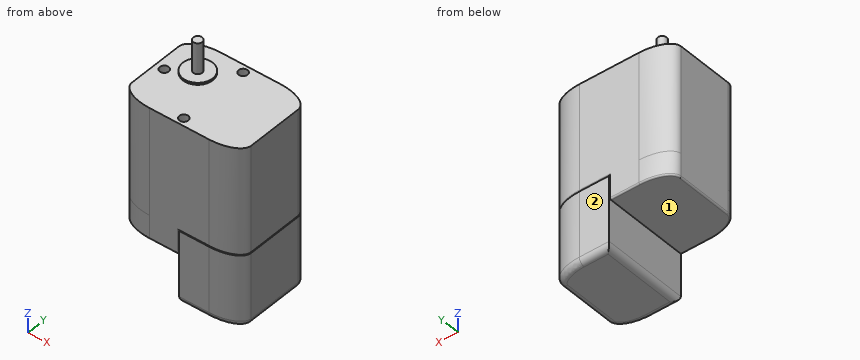
Autodesk Inventor part; units mm, degrees
ref_plane "YZ Plane" through (0, 0, 0) normal (1, 0, 0) x (0, 1, 0)
ref_plane "XZ Plane" through (0, 0, 0) normal (0, 1, 0) x (-1, 0, 0)
ref_plane "XY Plane" through (0, 0, 0) normal (0, 0, 1) x (1, 0, 0)
sketch "Sketch1" plane through (0, 0, 0) normal (0, 0, 1) x (1, 0, 0)
  ellipse E0 centre (10, 24) end of major axis (0, 24) minor radius 5 (10, 29) -> (0, 24) ccw
  ellipse E1 centre (30, 24) end of major axis (40, 24) minor radius 5 (40, 24) -> (30, 29) ccw
  ellipse E2 centre (30, 5) end of major axis (40, 5) minor radius 5 (30, 0) -> (40, 5) ccw
  ellipse E3 centre (10, 5) end of major axis (0, 5) minor radius 5 (0, 5) -> (10, 0) ccw
  line L0 (30, 29) -> (10, 29)
  line L1 (0, 24) -> (0, 5)
  line L2 (10, 0) -> (30, 0)
  line L3 (40, 5) -> (40, 24)
  point P0 (0, 0)
extrude "Extrusion2" add sketch "Sketch1" along normal blind 36
sketch "Sketch2" plane through (0, 0, 36) normal (0, 0, 1) x (1, 0, 0)
  line L0 (0, 24) -> (0, 5)
  line L1 (10, 0) -> (30, 0)
  line L2 (30, 29) -> (10, 29)
  line L3 (14.358, 14.5) -> (-3.5199, 14.5)
  circle A0 centre (3, 14.5) radius 1.5
  line L4 (21.3512, 2.5) -> (5.4191, 2.5)
  line L5 (21.3512, 26.5) -> (5.4191, 26.5)
  line L6 (19.5, 31.1643) -> (19.5, -4.236)
  circle A1 centre (19.5, 26.5) radius 1.5001
  circle A2 centre (19.5, 2.5) radius 1.5001
  point P0 (0, 0)
  dimension "d16" = 29
  dimension "d17" = 14.5
  dimension "d18" = 3
  dimension "d19" = 3
  dimension "d20" = 24
  dimension "d21" = 12
  dimension "d22" = 16.5
extrude "Extrusion3" cut sketch "Sketch2" against normal blind 5
thread "Thread1"
thread "Thread2"
thread "Thread3"
sketch "Sketch3" plane through (0, 0, 36) normal (0, 0, 1) x (1, 0, 0)
  line L0 (0, 24) -> (0, 5)
  line L1 (30, 29) -> (10, 29)
  line L2 (-1.3483, 17.5) -> (17.9999, 17.5)
  line L3 (12, 35.2177) -> (12, 13)
  circle A0 centre (10.5, 19) radius 1.5
  point P0 (0, 0)
  dimension "d31" = 11.5
  dimension "d32" = 12
  dimension "d33" = 3
  dimension "d34" = 1.5
  dimension "d35" = 1.5
extrude "Extrusion4" add sketch "Sketch3" along normal blind 11 contours A0
sketch "Sketch4" plane through (0, 0, 36) normal (0, 0, 1) x (1, 0, 0)
  circle A0 centre (10.5, 19) radius 1.5
  circle A1 centre (10.5, 19) radius 5
  point P0 (0, 0)
  dimension "d40" = 10
extrude "Extrusion5" add sketch "Sketch4" along normal blind 0.67
sketch "Sketch5" plane through (0, 0, 0) normal (0, 0, -1) x (-1, 0, 0)
  ellipse E0 centre (-10, 24) end of major axis (0, 24) minor radius 5 (0, 24) -> (-10, 29) ccw
  line L0 (-30, 29) -> (-10, 29)
  line L1 (-40, 5) -> (-40, 24)
  line L2 (-10, 0) -> (-30, 0)
  ellipse E1 centre (-10, 5) end of major axis (0, 5) minor radius 5 (-10, 0) -> (0, 5) ccw
  line L3 (0, 24) -> (0, 5)
  line L4 (-20, 29) -> (-20, 0)
  point P0 (0, 0)
  dimension "d42" = 40
  dimension "d43" = 20
extrude "Extrusion6" add sketch "Sketch5" along normal blind 8
sketch "Sketch6" plane through (0, 0, 0) normal (0, 0, -1) x (-1, 0, 0)
  line L0 (-20, 0) -> (-20, 29)
  line L1 (-30, 29) -> (-20, 29)
  ellipse E0 centre (-30, 24) end of major axis (-40, 24) minor radius 5 (-30, 29) -> (-40, 24) ccw
  line L2 (-40, 5) -> (-40, 24)
  ellipse E1 centre (-30, 5) end of major axis (-40, 5) minor radius 5 (-40, 5) -> (-30, 0) ccw
  line L3 (-20, 0) -> (-30, 0)
  point P0 (0, 0)
fillet "Fillet2" radius 0.5 13 edges at (15, 29, -8) (0, 14.5, -8) (2.9289, 1.4645, -8) (15, 0, -8) (2.9289, 27.5355, -8) (20, 29, -4) (37.0711, 27.5355, 0) (40, 14.5, 0) (37.0711, 1.4645, 0) (25, 0, 0) (25, 29, 0) (20, 14.5, -8) (20, 0, -4)
extrude "Extrusion8" add sketch "Sketch6" along normal blind 24
fillet "Fillet3" radius 2 6 edges at (25, 0, -24) (40, 14.5, -24) (37.0711, 27.5355, -24) (25, 29, -24) (37.0711, 1.4645, -24) (20, 14.5, -24)
properties part number "12V geared motor"
Could you check a few things on this model? Use its own coordinates, in mm. Face numbers are marked on the shaded views. A direction names the side the tool comes from. Coordinates: 2 decimals unless noted, no trailing zeros. Loops run counter-clockwise (first coordinate to the right, second up) from the corner with the lowest first, then second, coordinate; pieces in that order, holes last.
1) Will these pins go through, and if not, where does the flat tip stop? pin 1 Ø5 at (x, y) = (3, 14.5) entering from +Z; pin 2 Ø1 at (x, z) = (31.5, 12.5) entering from +Y; pin 3 Ø1 at (x, y) = (17.5, 6.5) entering from -Z.
Reported:
pin 1: stops at z = 36
pin 2: stops at y = 28.97
pin 3: stops at z = -8
2) Imagine slicing it at D-D (y = 22.5). List the corners of the cut face in (x, z) for me.
Reported:
outline: (0, -7.5) arc R0.5 ccw to (0.5, -8) - (19.5, -8) arc R0.5 ccw to (20, -7.5) - (20, -22) arc R2 ccw to (22, -24) - (38, -24) arc R2 ccw to (40, -22) - (40, 0) - (39.5, 0) arc R0.5 ccw to (40, 0.5) - (40, 36) - (14.07, 36) - (14.07, 36.67) - (6.93, 36.67) - (6.93, 36) - (0, 36) - close
3) Imagine slicing it at B-B (x = 24). List the corners of the cut face in (y, z) for me.
Reported:
outline: (0, -22) arc R2 ccw to (2, -24) - (27, -24) arc R2 ccw to (29, -22) - (29, 0) - (28.5, 0) arc R0.5 ccw to (29, 0.5) - (29, 36) - (0, 36) - (0, 0.5) arc R0.5 ccw to (0.5, 0) - (0, 0) - close
4) Which directions (+Z, -Z, +X, -X, +Y, -Y) give clear straight access to the entire face, cutting with the end or side of a thin tool? Please do the marked faces 1 and 2.
Reported:
face 1: -Z, -X, +Y, -Y
face 2: +Z, -Z, +X, -X, +Y
5) Please list where these lines run through material, in increasing order: line 1 along Y through (x, z) = (19.5, 32.9); line 2 along X through (y, z) = (14.5, 33.9); line 3 along Z through (x, y) = (7, 13).
Reported:
line 1: y = 0 to 1, 4 to 25, 28 to 29
line 2: x = 0 to 1.5, 4.5 to 40
line 3: z = -8 to 36
6) Imagine slicing it at A-A (y = 9.5). List the corners of the cut face in (x, z) for me, and give its area (3 significant figures).
Reported:
outline: (0, -7.5) arc R0.5 ccw to (0.5, -8) - (19.5, -8) arc R0.5 ccw to (20, -7.5) - (20, -22) arc R2 ccw to (22, -24) - (38, -24) arc R2 ccw to (40, -22) - (40, 0) - (39.5, 0) arc R0.5 ccw to (40, 0.5) - (40, 36) - (0, 36) - close
area: 2,080 mm2
7) Imagine slicing it at C-C (z = 38). List the corners of the cut face in (x, y) for me.
Reported:
outline: circle Ø3 at (10.5, 19)
